from build123d import *

# Parameters (mm, degrees)
SKETCH_1_R      = 2.5
SKETCH_1_R_2    = 1.5
SKETCH_1_R_3    = 19
EXTRUDE_1_DEPTH = 5
FILLET_1_R      = 5


with BuildPart() as part:
    # 草图1 → 凸台-拉伸1 (new body)
    with BuildSketch(Plane.XY):
        Polygon((-86, 75), (-86, -75), (86, -75), (111, -75), (111, 75), (111, 113), (-86, 113), align=None)
        with Locations((-73, 60)):
            Circle(SKETCH_1_R, mode=Mode.SUBTRACT)
        with Locations((-53, 60)):
            Circle(SKETCH_1_R, mode=Mode.SUBTRACT)
        with Locations((-73, 35)):
            Circle(SKETCH_1_R, mode=Mode.SUBTRACT)
        with Locations(Location((-53, 10, 0), (0, 0, 180))):
            Circle(SKETCH_1_R, mode=Mode.SUBTRACT)
        with Locations(Location((-73, 10, 0), (0, 0, 180))):
            Circle(SKETCH_1_R, mode=Mode.SUBTRACT)
        with Locations((75, 60)):
            Circle(SKETCH_1_R, mode=Mode.SUBTRACT)
        with Locations((75, 35)):
            Circle(SKETCH_1_R, mode=Mode.SUBTRACT)
        with Locations((75, 10)):
            Circle(SKETCH_1_R, mode=Mode.SUBTRACT)
        with Locations((55, 60)):
            Circle(SKETCH_1_R, mode=Mode.SUBTRACT)
        with Locations((55, 35)):
            Circle(SKETCH_1_R, mode=Mode.SUBTRACT)
        with Locations((55, 10)):
            Circle(SKETCH_1_R, mode=Mode.SUBTRACT)
        with Locations((-53, 35)):
            Circle(SKETCH_1_R, mode=Mode.SUBTRACT)
        with Locations((100, 60)):
            Circle(SKETCH_1_R, mode=Mode.SUBTRACT)
        with Locations((100, 35)):
            Circle(SKETCH_1_R, mode=Mode.SUBTRACT)
        with Locations((100, 10)):
            Circle(SKETCH_1_R, mode=Mode.SUBTRACT)
        with Locations((-8.5, 99)):
            Circle(SKETCH_1_R_2, mode=Mode.SUBTRACT)
        with Locations((16.181724008, 84.75)):
            Circle(SKETCH_1_R_2, mode=Mode.SUBTRACT)
        with Locations((16.181724008, 56.25)):
            Circle(SKETCH_1_R_2, mode=Mode.SUBTRACT)
        with Locations((-8.5, 42)):
            Circle(SKETCH_1_R_2, mode=Mode.SUBTRACT)
        with Locations((-33.181724008, 56.25)):
            Circle(SKETCH_1_R_2, mode=Mode.SUBTRACT)
        with Locations((-33.181724008, 84.75)):
            Circle(SKETCH_1_R_2, mode=Mode.SUBTRACT)
        with Locations((-8.5, 70.5)):
            Circle(SKETCH_1_R_3, mode=Mode.SUBTRACT)
        with BuildLine():
            Line((55, -15.5), (60, -15.5))
            ThreePointArc((60, -15.5), (62.5, -18), (60, -20.5))
            Line((60, -20.5), (55, -20.5))
            ThreePointArc((55, -20.5), (52.5, -18), (55, -15.5))
        make_face(mode=Mode.SUBTRACT)
        with BuildLine():
            Line((55, -57.5), (60, -57.5))
            ThreePointArc((60, -57.5), (62.5, -60), (60, -62.5))
            Line((60, -62.5), (55, -62.5))
            ThreePointArc((55, -62.5), (52.5, -60), (55, -57.5))
        make_face(mode=Mode.SUBTRACT)
        with BuildLine():
            Line((97, -15.5), (102, -15.5))
            ThreePointArc((102, -15.5), (104.5, -18), (102, -20.5))
            Line((102, -20.5), (97, -20.5))
            ThreePointArc((97, -20.5), (94.5, -18), (97, -15.5))
        make_face(mode=Mode.SUBTRACT)
        with BuildLine():
            Line((97, -57.5), (102, -57.5))
            ThreePointArc((102, -57.5), (104.5, -60), (102, -62.5))
            Line((102, -62.5), (97, -62.5))
            ThreePointArc((97, -62.5), (94.5, -60), (97, -57.5))
        make_face(mode=Mode.SUBTRACT)
        with BuildLine():
            Line((-73, -15), (17, -15))
            ThreePointArc((17, -15), (20, -18), (17, -21))
            Line((17, -21), (-73, -21))
            ThreePointArc((-73, -21), (-76, -18), (-73, -15))
        make_face(mode=Mode.SUBTRACT)
        with BuildLine():
            Line((-73, -57), (17, -57))
            ThreePointArc((17, -57), (20, -60), (17, -63))
            Line((17, -63), (-73, -63))
            ThreePointArc((-73, -63), (-76, -60), (-73, -57))
        make_face(mode=Mode.SUBTRACT)
        with BuildLine():
            Line((-73, -29), (17, -29))
            ThreePointArc((17, -29), (20, -32), (17, -35))
            Line((17, -35), (-73, -35))
            ThreePointArc((-73, -35), (-76, -32), (-73, -29))
        make_face(mode=Mode.SUBTRACT)
        with BuildLine():
            Line((-73, -43), (17, -43))
            ThreePointArc((17, -43), (20, -46), (17, -49))
            Line((17, -49), (-73, -49))
            ThreePointArc((-73, -49), (-76, -46), (-73, -43))
        make_face(mode=Mode.SUBTRACT)
        with BuildLine():
            Line((100, 102), (30, 102))
            ThreePointArc((30, 102), (27, 105), (30, 108))
            Line((30, 108), (100, 108))
            ThreePointArc((100, 108), (103, 105), (100, 102))
        make_face(mode=Mode.SUBTRACT)
        with BuildLine():
            Line((100, 88), (30, 88))
            ThreePointArc((30, 88), (27, 91), (30, 94))
            Line((30, 94), (100, 94))
            ThreePointArc((100, 94), (103, 91), (100, 88))
        make_face(mode=Mode.SUBTRACT)
        with BuildLine():
            Line((102, -35), (32, -35))
            ThreePointArc((32, -35), (29, -32), (32, -29))
            Line((32, -29), (102, -29))
            ThreePointArc((102, -29), (105, -32), (102, -35))
        make_face(mode=Mode.SUBTRACT)
        with BuildLine():
            Line((102, -49), (32, -49))
            ThreePointArc((32, -49), (29, -46), (32, -43))
            Line((32, -43), (102, -43))
            ThreePointArc((102, -43), (105, -46), (102, -49))
        make_face(mode=Mode.SUBTRACT)
    extrude(amount=EXTRUDE_1_DEPTH)

    # 圆角1
    fillet_1_edges = [part.edges().sort_by_distance(p)[0] for p in [
        (-86, 113, 2.5),
        (111, 113, 2.5),
        (111, -75, 2.5),
        (-86, -75, 2.5),
    ]]
    fillet(fillet_1_edges, radius=FILLET_1_R)


solid = part.part
The model under review builds one solid part; all positions refer to its coordinate system, in mm. Round coordinates to 2 decimals unless told otherwise and drop trailing zeros. Loops run counter-clockwise (first coordinate to the right, second up) from the corner with the lowest first, then second, coordinate; pieces in that order, holes last. Notation, with made-up numbers: (14.25, 72) -> (73.25, 72) arc R13 ccw to (73.25, 92) -> close; hole circle Ø2 at (80, 60). An arc over 180 degrees is marked (long way). Answer as CSV lines item,"result".
1) Draft analysis for pull direction X (two halves, no side actions). For faces 1 (the face through (-27, -63, 2)), 2 (the face through (111, 18, 2)), state which applies: pulls with the +X half, pulls with the -X half, needs draft (parallel to the pull), parting line crosses it, or undercut.
Geometry results:
face 1,"undercut"
face 2,"pulls with the +X half"
2) To check wall thickness, follow line 1 along Y through (x, z) = (81, 4.6); line 2 along Y through (x, z) = (-61, 1.7); line 3 along X through (y, z) = (85.5, 2.6). State the ranges of each line that lie inside material, in increasing order. Write a range as from..to.
Geometry results:
line 1,"y = -75..-49, -43..-35, -29..88, 94..102, 108..113"
line 2,"y = -75..-63, -57..-49, -43..-35, -29..-21, -15..113"
line 3,"x = -86..-34.48, -31.88..-20.16, 3.16..14.88, 17.48..111"
3) Add section A-A on x = -53. State how many separate pieces and enclosed holes the cut face has, plus the area to 3 significant figures.
Geometry results:
separate pieces,"8"
enclosed holes,"0"
area,"745 mm²"
4) Add section C-C on x = 70. Write out the cut boundary in (y, z), plus the area to 3 significant figures.
Geometry results:
outline,"(-75, 0) -> (-49, 0) -> (-49, 5) -> (-75, 5) -> close; (-43, 0) -> (-35, 0) -> (-35, 5) -> (-43, 5) -> close; (-29, 0) -> (88, 0) -> (88, 5) -> (-29, 5) -> close; (94, 0) -> (102, 0) -> (102, 5) -> (94, 5) -> close; (108, 0) -> (113, 0) -> (113, 5) -> (108, 5) -> close"
area,"820 mm²"
5) Add section B-B on y = 105. Write out the cut boundary in (x, z).
Geometry results:
outline,"(-86, 0) -> (27, 0) -> (27, 5) -> (-86, 5) -> close; (103, 0) -> (111, 0) -> (111, 5) -> (103, 5) -> close"
6) Add section D-D on y = -18. Write out the cut boundary in (x, z).
Geometry results:
outline,"(-86, 0) -> (-76, 0) -> (-76, 5) -> (-86, 5) -> close; (20, 0) -> (52.5, 0) -> (52.5, 5) -> (20, 5) -> close; (62.5, 0) -> (94.5, 0) -> (94.5, 5) -> (62.5, 5) -> close; (104.5, 0) -> (111, 0) -> (111, 5) -> (104.5, 5) -> close"
